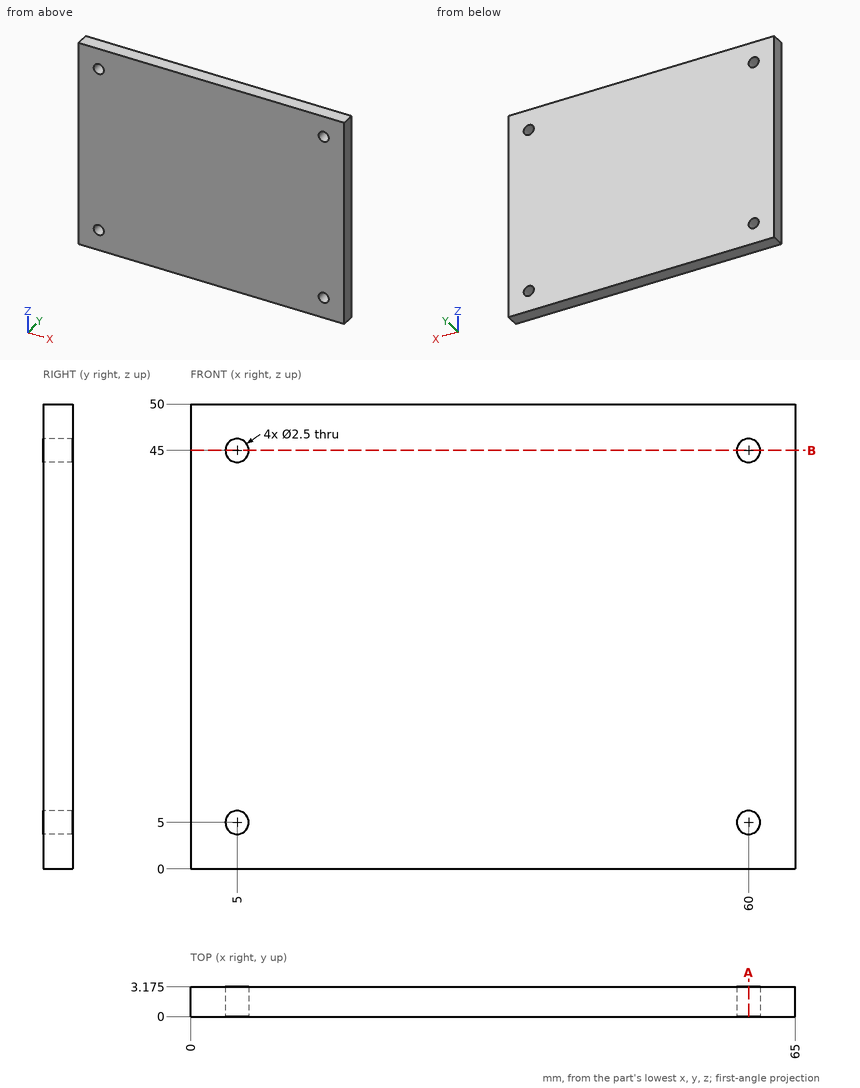
Study the drawing (mm; zero at the part's minimum x, y, z) and answer. Coordinates: 2 decimals unless noted, no trailing zeros. Write each loop counter-clockwise with the first axis right and the second up, starting at its lowest first coordinate (ties: lowest second). Pieces come first, ordered by that corner, then holes. Notation, with made-up numbers: (56.25, -23.5) - (97.25, -23.5) arc R36 cw to (97.25, 10.5) - close; hole circle Ø6 at (46.25, -9.5). An arc over 180 degrees is marked (long way). Answer as a JSON object with one key per item and string values.
Q1. Find section A-A (x = 60). Write down the section's boundary in (y, z) (3 decimals).
Results list:
{"outline": "(0, 0) - (3.175, 0) - (3.175, 3.75) - (0, 3.75) - close; (0, 6.25) - (3.175, 6.25) - (3.175, 43.75) - (0, 43.75) - close; (0, 46.25) - (3.175, 46.25) - (3.175, 50) - (0, 50) - close"}
Q2. Find section B-B (z = 45). Write down the section's boundary in (x, y) (3 decimals), plus the area to 4 significant figures.
Results list:
{"outline": "(0, 0) - (3.75, 0) - (3.75, 3.175) - (0, 3.175) - close; (6.25, 0) - (58.75, 0) - (58.75, 3.175) - (6.25, 3.175) - close; (61.25, 0) - (65, 0) - (65, 3.175) - (61.25, 3.175) - close", "area": "190.5 mm^2"}
Q3. Consider L1, parallel to Z at x = 5, y = 1.7; L2, parallel to X at y = 2.3, z = 44. Determine where each line is inside the solid, lowest interval first. Write a range as from..to.
Results list:
{"L1": "z = 0..3.75, 6.25..43.75, 46.25..50", "L2": "x = 0..4.25, 5.75..59.25, 60.75..65"}
Q4. Given pin 1 Ø4 at (x, z) = (60, 45) entering from +Y (3 decimals); pin 2 Ø2 at (x, z) = (60, 5) entering from -Y, each flat-ended and moving along its own axis, determine where each tip first touches the part or whether it passes through.
Results list:
{"pin 1": "stops at y = 3.175", "pin 2": "passes through"}
